For this review, use the dimensioned drawing (mm, ordinates from the lowest corner) and the shaded views. Give positions to 0.01 mm unless a question says otherwise; leave off trailing zeros. Write each loop counter-clockwise with the first axis right and the second up, starting at its lowest first coordinate (ties: lowest second). Pieces come first, ordered by that corner, then holes.
1) We need section B-B on z = 25. Give the boundary of the cut face in (x, y), and give its area (3 significant figures).
2) We need section C-C on y = 7.25. Give the boundary of the cut face in (x, z), and give its area (3 significant figures).
3) Wall thickness on line 1 along X through (y, z) = (13.5, 25); line 2 along X through (y, z) = (5, 12.5): over which ranges is each line inside the solid? List them lowest first.
4) We need section D-D on z = 46. Give the boundary of the cut face in (x, y), and give its area (3 significant figures).
5) Draft analysis for pull direction X (two halves, no side actions). For the marked faces 1, 2 and 3, state which applies: pulls with the +X half, pulls with the -X half, needs draft (parallel to the pull), parting line crosses it, or undercut.
6) We need section A-A on x = 25. Give the boundary of the cut face in (y, z), and give its area (3 significant figures).
7) For P1, Ø3, axis at y = 6, z = 27, coming from the -X side (3 decimals); P2, Ø1, axis at y = 17, z = 18, coming from the +X side; P3, Ø8, axis at x = 18, y = 12, coming from the +Z side, all flat-tipped, find the tip position at first contact; note any pin that passes through.
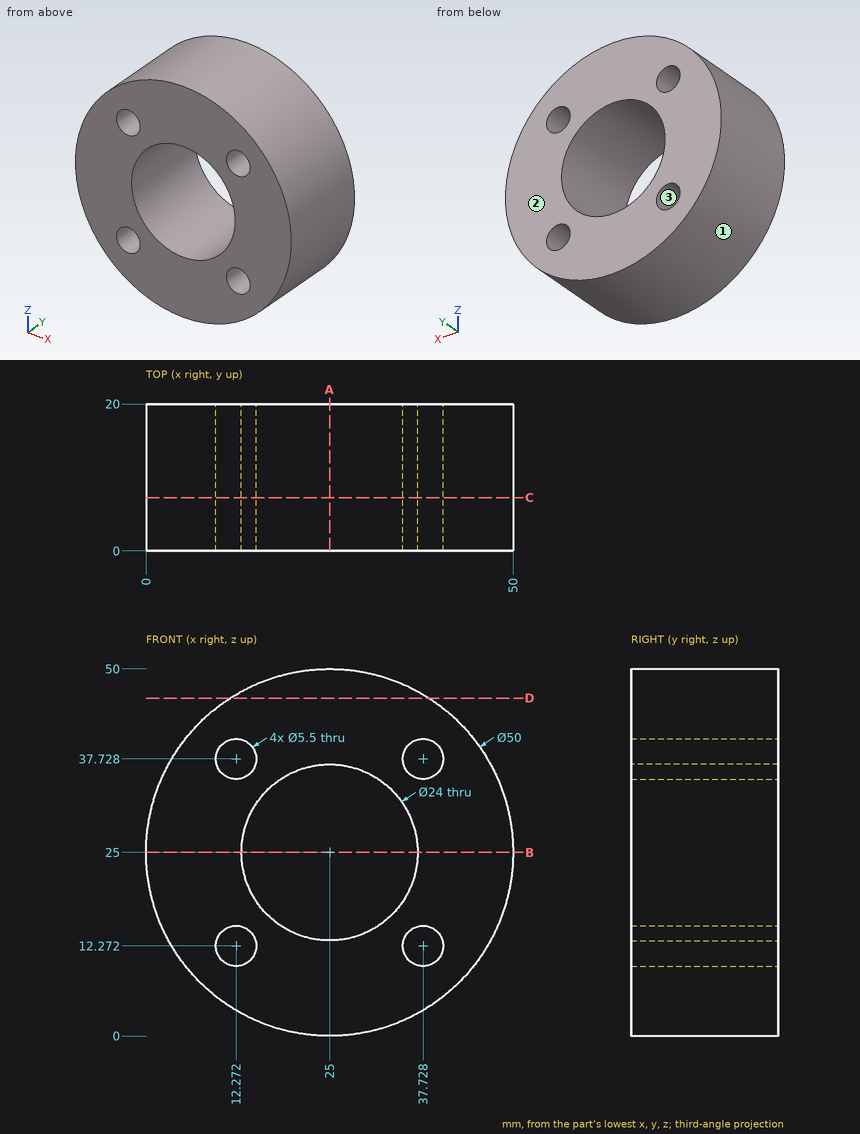
Results list:
1. outline: (0, 0) - (13, 0) - (13, 20) - (0, 20) - close; (37, 0) - (50, 0) - (50, 20) - (37, 20) - close
1. area: 520 mm2
2. outline: circle Ø50 at (25, 25); hole circle Ø5.5 at (12.27, 12.27); hole circle Ø5.5 at (12.27, 37.73); hole circle Ø24 at (25, 25); hole circle Ø5.5 at (37.73, 12.27); hole circle Ø5.5 at (37.73, 37.73)
2. area: 1,420 mm2
3. line 1: x = 0 to 13, 37 to 50
3. line 2: x = 3.35 to 9.53, 15.01 to 34.99, 40.47 to 46.65
4. outline: (11.44, 0) - (38.56, 0) - (38.56, 20) - (11.44, 20) - close
4. area: 543 mm2
5. face 1: parting line crosses it
5. face 2: needs draft
5. face 3: undercut
6. outline: (0, 0) - (20, 0) - (20, 13) - (0, 13) - close; (0, 37) - (20, 37) - (20, 50) - (0, 50) - close
6. area: 520 mm2
7. P1: stops at x = 0.005
7. P2: stops at x = 49.14
7. P3: stops at z = 49.82
